Could you check a few things on this drawing? It's one solid part, dimensions in mm from its lowest x, y, z. A direction names the side the tool comes from. Coordinates: 2 decimals unless noted, no trailing zeros. Write each loop counter-clockwise with the first axis right and the second up, starting at its lowest first coordinate (ties: lowest second). Pieces come first, ordered by that corner, then holes.
Item 1: Please list where these lines run through material, in increasing order: line 1 (Z direction, x = 4, y = 12.5); line 2 (Y direction, x = 8.75, z = 14); line 3 (Z direction, x = 14, y = 2.75).
Item 2: I'm going to push flat-ended pins straight in: P1, Ø5, axis at y = 13.5, z = 18, coming from the -X side; P2, Ø4, axis at x = 8, z = 17.5, coming from the -Y side; P3, Ø1.5, axis at y = 5, z = 22, coming from the +X side. Where does each tip first touch, or does it pass through?
Item 3: For the marked faces 4, 5 and 6, which set-ups out of +Z, -Z, +X, -X, +Y, -Y let a thin tool reach every point of the face, with its end or its side?
Item 4: If we mould it in two halves opening along Y, with no side actions, what happens to the marked faces 1, 2 and 3? For each: pulls with the +Y half, pulls with the -Y half, needs draft (parallel to the pull), parting line crosses it, or undercut.
Item 5: I want a section at C-C (z = 8.5). Please give me the cut outline in (x, y), and give its area (3 significant figures).
Item 6: I want a section at A-A (y = 8). Please give me the cut outline in (x, z), and give its area (3 significant figures).
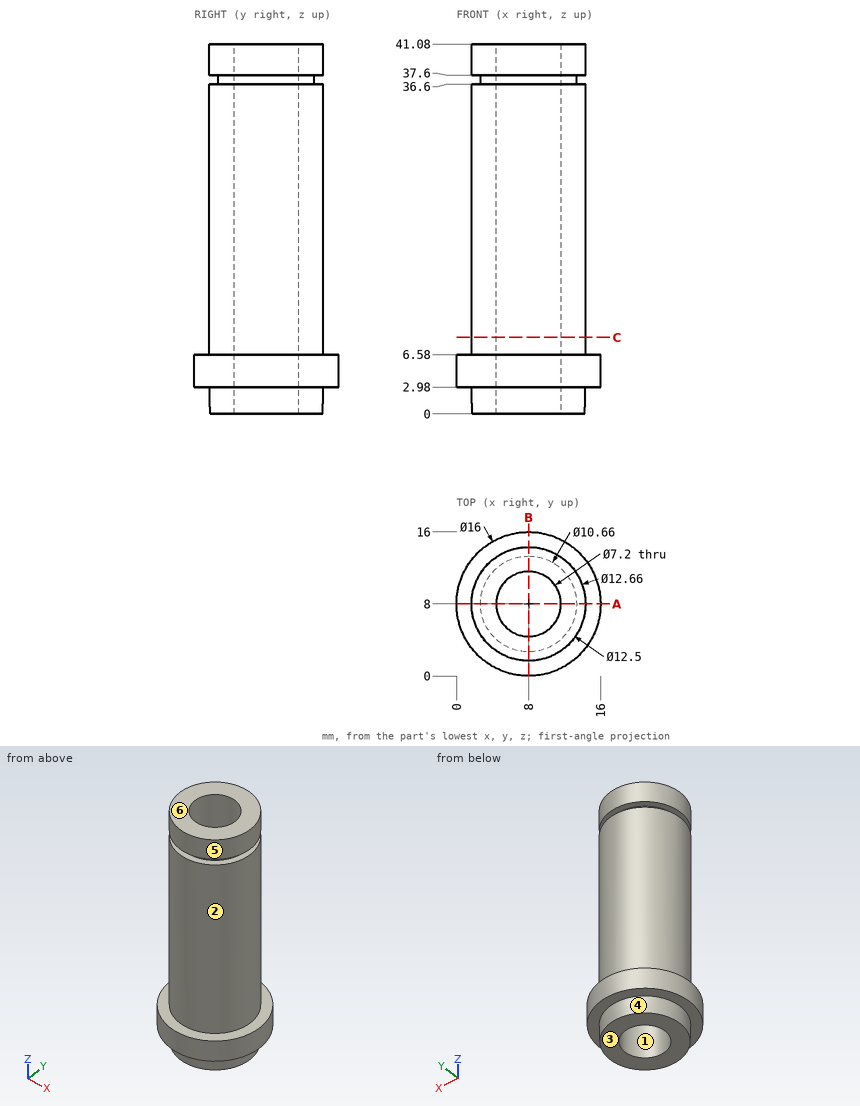
Answer:
1. line 1: z = 0 to 36.6, 37.6 to 41.08
1. line 2: y = 1.71 to 4.48, 11.52 to 14.29
1. line 3: z = 2.98 to 6.58
2. P1: stops at x = 2.43
2. P2: stops at y = 1.67
2. P3: stops at x = 13.92
3. face 4: -Z
3. face 5: +Z
3. face 6: +Z, +X, -X, +Y, -Y
4. face 1: undercut
4. face 2: parting line crosses it
4. face 3: needs draft
5. outline: circle Ø12.66 at (8, 8); hole circle Ø7.2 at (8, 8)
5. area: 85.2 mm2
6. outline: (0, 2.98) - (1.67, 2.98) - (1.75, 0) - (4.4, 0) - (4.4, 41.08) - (1.67, 41.08) - (1.67, 37.6) - (2.67, 37.6) - (2.67, 36.6) - (1.67, 36.6) - (1.67, 6.58) - (0, 6.58) - close; (11.6, 0) - (14.25, 0) - (14.33, 2.98) - (16, 2.98) - (16, 6.58) - (14.33, 6.58) - (14.33, 36.6) - (13.33, 36.6) - (13.33, 37.6) - (14.33, 37.6) - (14.33, 41.08) - (11.6, 41.08) - close
6. area: 234 mm2
